Read the model definition and answer for the solid it produces. Units are mm, in the model's axes. A direction names the side the tool comes from. Coordinates: 2 decimals unless noted, no trailing zeros. Loops run counter-clockwise (first coordinate to the right, second up) from the corner with the lowest first, then second, coordinate; pieces in that order, holes last. Notation, with made-up numbers: (62.5, -2.5) -> (118.5, -2.5) arc R29 ccw to (118.5, 28.5) -> close; hole circle Ø2 at (67.25, 18.5). An arc over 180 degrees is marked (long way). Answer in a Markdown table with one row per item.
```python
from build123d import *

# Parameters (mm, degrees)
SKETCH_1_W           = 100
SKETCH_1_H           = 100
EXTRUDE_1_DEPTH      = 4
SKETCH_2_R           = 2.15
CUT_EXTRUDE_1_DEPTH  = 142.477913471
SKETCH_3_R           = 1.65
CUT_EXTRUDE_2_DEPTH  = 142.477913471
SKETCH_4_R           = 1.65
CUT_EXTRUDE_3_DEPTH  = 142.477913471
SKETCH_5_W           = 20.5
SKETCH_5_H           = 41.5
CUT_EXTRUDE_4_DEPTH  = 10
SKETCH_6_W           = 55
SKETCH_6_H           = 100
CUT_EXTRUDE_5_DEPTH  = 10
FILLET_2_R           = 1.2
SKETCH_8_R           = 1.65
CUT_EXTRUDE_6_DEPTH  = 142.477913471
SKETCH_9_W           = 15.75
SKETCH_9_H           = 78.5
CUT_EXTRUDE_7_DEPTH  = 142.477913471
CUT_EXTRUDE_8_DEPTH  = 10
FILLET_5_R           = 3
SKETCH_11_W          = 29.25
SKETCH_11_H          = 14
CUT_EXTRUDE_9_DEPTH  = 10
FILLET_7_R           = 3
SKETCH_12_R          = 1.65
CUT_EXTRUDE_10_DEPTH = 10
FILLET_8_R           = 3
EXTRUDE_2_DEPTH      = 4
FILLET_9_R           = 5
CUT_EXTRUDE_11_DEPTH = 10
FILLET_10_R          = 1.7
SKETCH_15_R          = 1.65
CUT_EXTRUDE_12_DEPTH = 10
FILLET_11_R          = 5


with BuildPart() as part:
    # 草图1 → 凸台-拉伸1 (new body)
    with BuildSketch(Plane.XY):
        with Locations((50, -50)):
            Rectangle(SKETCH_1_W, SKETCH_1_H)
    extrude(amount=EXTRUDE_1_DEPTH)

    # 草图2 → 切除-拉伸1 (cut, through all)
    with BuildSketch(Plane.XY.offset(4)):
        with Locations((80, -66)):
            Circle(SKETCH_2_R)
        with Locations((90, -66)):
            Circle(SKETCH_2_R)
        with Locations((90, -18)):
            Circle(SKETCH_2_R)
        with Locations((80, -18)):
            Circle(SKETCH_2_R)
    extrude(amount=-CUT_EXTRUDE_1_DEPTH, mode=Mode.SUBTRACT)

    # 草图3 → 切除-拉伸2 (cut, through all)
    with BuildSketch(Plane.XY.offset(4)):
        with Locations((73, -95)):
            Circle(SKETCH_3_R)
        with Locations((73, -85)):
            Circle(SKETCH_3_R)
        with Locations((85, -85)):
            Circle(SKETCH_3_R)
        with Locations((85, -95)):
            Circle(SKETCH_3_R)
    extrude(amount=-CUT_EXTRUDE_2_DEPTH, mode=Mode.SUBTRACT)

    # 草图4 → 切除-拉伸3 (cut, through all)
    with BuildSketch(Plane.XY.offset(4)):
        with BuildLine():
            ThreePointArc((81, -100), (71.5, -90.5), (62, -100))
            Line((62, -100), (81, -100))
        make_face()
        with Locations((73, -95)):
            Circle(SKETCH_4_R, mode=Mode.SUBTRACT)
    extrude(amount=-CUT_EXTRUDE_3_DEPTH, mode=Mode.SUBTRACT)

    # 草图5 → 切除-拉伸4 (cut)
    with BuildSketch(Plane.XY.offset(4)):
        with Locations((85, -42)):
            Rectangle(SKETCH_5_W, SKETCH_5_H)
    extrude(amount=-CUT_EXTRUDE_4_DEPTH, mode=Mode.SUBTRACT)

    # 草图6 → 切除-拉伸5 (cut)
    with BuildSketch(Plane.XY.offset(4)):
        with Locations((27.5, -50)):
            Rectangle(SKETCH_6_W, SKETCH_6_H)
    extrude(amount=-CUT_EXTRUDE_5_DEPTH, mode=Mode.SUBTRACT)

    # 圆角2
    fillet_2_edges = [part.edges().sort_by_distance(p)[0] for p in [
        (95.25, -62.75, 2),
        (74.75, -62.75, 2),
        (74.75, -21.25, 2),
        (95.25, -21.25, 2),
    ]]
    fillet(fillet_2_edges, radius=FILLET_2_R)

    # 草图8 → 切除-拉伸6 (cut, through all)
    with BuildSketch(Plane.XY.offset(4)):
        with Locations((59, -85)):
            Circle(SKETCH_8_R)
    extrude(amount=-CUT_EXTRUDE_6_DEPTH, mode=Mode.SUBTRACT)

    # 草图9 → 切除-拉伸7 (cut, through all)
    with BuildSketch(Plane.XY.offset(4)):
        with BuildLine():
            Line((71.5, -90.5), (55, -90.5))
            Line((55, -90.5), (55, -100))
            Line((55, -100), (62, -100))
            ThreePointArc((62, -100), (64.782485579, -93.282485579), (71.5, -90.5))
        make_face()
        with Locations((62.875, -39.25)):
            Rectangle(SKETCH_9_W, SKETCH_9_H)
    extrude(amount=-CUT_EXTRUDE_7_DEPTH, mode=Mode.SUBTRACT)

    # 草图10 → 切除-拉伸8 (cut)
    with BuildSketch(Plane.XY.offset(4)):
        with BuildLine():
            Line((100, -87.5), (55, -87.5))
            Line((55, -87.5), (55, -90.5))
            Line((55, -90.5), (71.5, -90.5))
            ThreePointArc((71.5, -90.5), (78.217514421, -93.282485579), (81, -100))
            Line((81, -100), (100, -100))
            Line((100, -100), (100, -87.5))
        make_face()
    extrude(amount=-CUT_EXTRUDE_8_DEPTH, mode=Mode.SUBTRACT)

    # 圆角5
    fillet_5_edges = [part.edges().sort_by_distance(p)[0] for p in [
        (100, -87.5, 2),
        (55, -87.5, 2),
    ]]
    fillet(fillet_5_edges, radius=FILLET_5_R)

    # 草图11 → 切除-拉伸9 (cut)
    with BuildSketch(Plane.XY.offset(4)):
        with Locations((85.375, -7)):
            Rectangle(SKETCH_11_W, SKETCH_11_H)
    extrude(amount=-CUT_EXTRUDE_9_DEPTH, mode=Mode.SUBTRACT)

    # 圆角7
    fillet_7_edges = [part.edges().sort_by_distance(p)[0] for p in [
        (70.75, -14, 2),
        (100, -14, 2),
    ]]
    fillet(fillet_7_edges, radius=FILLET_7_R)

    # 草图12 → 切除-拉伸10 (cut)
    with BuildSketch(Plane.XY.offset(4)):
        with BuildLine():
            Line((64.339745962, -87.5), (81.660254038, -87.5))
            ThreePointArc((81.660254038, -87.5), (73, -82.5), (64.339745962, -87.5))
        make_face()
        with Locations((73, -85)):
            Circle(SKETCH_12_R, mode=Mode.SUBTRACT)
    extrude(amount=-CUT_EXTRUDE_10_DEPTH, mode=Mode.SUBTRACT)

    # 圆角8
    fillet_8_edges = [part.edges().sort_by_distance(p)[0] for p in [
        (64.339745962, -87.5, 2),
        (81.660254038, -87.5, 2),
    ]]
    fillet(fillet_8_edges, radius=FILLET_8_R)

    # 草图13 → 凸台-拉伸2 (add)
    with BuildSketch(Plane.XY.offset(4)):
        Polygon((70.75, -51.220199781), (55, -78.5), (70.75, -78.5), align=None)
    extrude(amount=-EXTRUDE_2_DEPTH)

    # 圆角9
    fillet_9_edges = [part.edges().sort_by_distance(p)[0] for p in [
        (55, -78.5, 2),
        (70.75, -51.220199781, 2),
    ]]
    fillet(fillet_9_edges, radius=FILLET_9_R)

    # 草图14 → 切除-拉伸11 (cut)
    with BuildSketch(Plane.XY.offset(4)):
        Polygon((72.044228634, -79.339745962), (72.044228634, -56.97853003), (59.133974596, -79.339745962), align=None)
    extrude(amount=-CUT_EXTRUDE_11_DEPTH, mode=Mode.SUBTRACT)

    # 圆角10
    fillet_10_edges = [part.edges().sort_by_distance(p)[0] for p in [
        (72.044228634, -79.339745962, 2),
        (59.133974596, -79.339745962, 2),
        (72.044228634, -56.97853003, 2),
    ]]
    fillet(fillet_10_edges, radius=FILLET_10_R)

    # 草图15 → 切除-拉伸12 (cut)
    # profile 1 of 4: a face of its own
    with BuildSketch(Plane(origin=(0, 0, 0), x_dir=(-1, 0, 0), z_dir=(0, 0, -1))):
        with BuildLine():
            Line((-59.474464586, -70.75), (-55.667552662, -70.75))
            Line((-55.667552662, -70.75), (-55.667552662, -49.880453819))
            Line((-55.667552662, -49.880453819), (-70.75, -49.880453819))
            ThreePointArc((-70.75, -49.880453819), (-70.579629131, -51.174549044), (-70.080127019, -52.380453819))
            Line((-70.080127019, -52.380453819), (-59.474464586, -70.75))
        make_face()
    # profile 2 of 4: a face of its own
    with BuildSketch(Plane(origin=(0, 0, 0), x_dir=(-1, 0, 0), z_dir=(0, 0, -1))):
        with BuildLine():
            Line((-41.658398954, -70.75), (-55.667552662, -70.75))
            Line((-55.667552662, -70.75), (-59.474464586, -70.75))
            Line((-59.474464586, -70.75), (-55.669872981, -77.339745962))
            ThreePointArc((-55.669872981, -77.339745962), (-55.170370869, -78.545650737), (-55, -79.839745962))
            Line((-55, -79.839745962), (-55, -84.5))
            ThreePointArc((-55, -84.5), (-55.878679656, -86.621320344), (-58, -87.5))
            Line((-58, -87.5), (-62.753049234, -87.5))
            ThreePointArc((-62.753049234, -87.5), (-64.068636263, -87.196151103), (-65.11773018, -86.346153846))
            ThreePointArc((-65.11773018, -86.346153846), (-73, -82.5), (-80.88226982, -86.346153846))
            ThreePointArc((-80.88226982, -86.346153846), (-81.931363737, -87.196151103), (-83.246950766, -87.5))
            Line((-83.246950766, -87.5), (-97, -87.5))
            ThreePointArc((-97, -87.5), (-99.121320344, -86.621320344), (-100, -84.5))
            Line((-100, -84.5), (-100, -90.078728051))
            Line((-100, -90.078728051), (-41.658398954, -90.078728051))
            Line((-41.658398954, -90.078728051), (-41.658398954, -70.75))
        make_face()
    # profile 3 of 4: a face of its own
    with BuildSketch(Plane(origin=(0, 0, 0), x_dir=(-1, 0, 0), z_dir=(0, 0, -1))):
        with BuildLine():
            Line((-55.669872981, -77.339745962), (-59.474464586, -70.75))
            Line((-59.474464586, -70.75), (-64.09326674, -70.75))
            Line((-64.09326674, -70.75), (-60.606217783, -76.789745962))
            ThreePointArc((-60.606217783, -76.789745962), (-60.606217783, -78.489745962), (-62.078460969, -79.339745962))
            Line((-62.078460969, -79.339745962), (-70.344228634, -79.339745962))
            ThreePointArc((-70.344228634, -79.339745962), (-71.546310162, -78.84182749), (-72.044228634, -77.639745962))
            Line((-72.044228634, -77.639745962), (-72.044228634, -70.75))
            Line((-72.044228634, -70.75), (-100, -70.75))
            Line((-100, -70.75), (-100, -84.5))
            ThreePointArc((-100, -84.5), (-99.121320344, -86.621320344), (-97, -87.5))
            Line((-97, -87.5), (-83.246950766, -87.5))
            ThreePointArc((-83.246950766, -87.5), (-81.931363737, -87.196151103), (-80.88226982, -86.346153846))
            ThreePointArc((-80.88226982, -86.346153846), (-73, -82.5), (-65.11773018, -86.346153846))
            ThreePointArc((-65.11773018, -86.346153846), (-64.068636263, -87.196151103), (-62.753049234, -87.5))
            Line((-62.753049234, -87.5), (-58, -87.5))
            ThreePointArc((-58, -87.5), (-55.878679656, -86.621320344), (-55, -84.5))
            Line((-55, -84.5), (-55, -79.839745962))
            ThreePointArc((-55, -79.839745962), (-55.170370869, -78.545650737), (-55.669872981, -77.339745962))
        make_face()
        with Locations((-85, -85)):
            Circle(SKETCH_15_R, mode=Mode.SUBTRACT)
        with Locations((-59, -85)):
            Circle(SKETCH_15_R, mode=Mode.SUBTRACT)
    # profile 4 of 4: a face of its own
    with BuildSketch(Plane(origin=(0, 0, 0), x_dir=(-1, 0, 0), z_dir=(0, 0, -1))):
        with BuildLine():
            Line((-64.09326674, -70.75), (-59.474464586, -70.75))
            Line((-59.474464586, -70.75), (-70.080127019, -52.380453819))
            ThreePointArc((-70.080127019, -52.380453819), (-70.579629131, -51.174549044), (-70.75, -49.880453819))
            Line((-70.75, -49.880453819), (-70.75, -61.672153114))
            ThreePointArc((-70.75, -61.672153114), (-69.677380797, -61.759266435), (-68.871985448, -62.473016403))
            Line((-68.871985448, -62.473016403), (-64.09326674, -70.75))
        make_face()
    extrude(amount=-CUT_EXTRUDE_12_DEPTH, mode=Mode.SUBTRACT)

    # 圆角11
    fillet_11_edges = [part.edges().sort_by_distance(p)[0] for p in [
        (70.75, -61.672153114, 2),
        (100, -70.75, 2),
        (72.044228634, -70.75, 2),
    ]]
    fillet(fillet_11_edges, radius=FILLET_11_R)


solid = part.part
```
1. A cutting plane is placed at A-A on y = -18. Give the vertices of the cut face in (x, z).
A:
| item | result |
|---|---|
| outline | (70.75, 0) -> (77.85, 0) -> (77.85, 4) -> (70.75, 4) -> close; (82.15, 0) -> (87.85, 0) -> (87.85, 4) -> (82.15, 4) -> close; (92.15, 0) -> (100, 0) -> (100, 4) -> (92.15, 4) -> close |
2. Find the intervals of material crossed by probe 1 along Y at (x, z) = (80, 2.6); probe 2 along X at (y, z) = (-55, 2.2); probe 3 along Y at (x, z) = (87, 1.85), in increasing order.
A:
| item | result |
|---|---|
| probe 1 | y = -70.75 to -68.15, -63.85 to -62.75, -21.25 to -20.15, -15.85 to -14 |
| probe 2 | x = 70.75 to 74.75, 95.25 to 100 |
| probe 3 | y = -70.75 to -62.75, -21.25 to -14 |
3. The mould has two halves that part along Y. Classify faces 1 (the cylindrical face through (98.57, -69.25, 2.03)), 2 (the cylindrical face through (71.61, -14.9, 1.97)), 3 (the flat face through (74, -44, 0)), 4 (the cylindrical face through (75.092, -21.611, 1.972)): pulls with the +Y half, pulls with the -Y half, needs draft (parallel to the pull), parting line crosses it, or undercut.
A:
| item | result |
|---|---|
| face 1 | pulls with the -Y half |
| face 2 | pulls with the +Y half |
| face 3 | needs draft |
| face 4 | undercut |
4. A cutting plane is placed at B-B on x = 85.5. Give the vertices of the cut face in (y, z), and give its area (3 significant figures).
A:
| item | result |
|---|---|
| outline | (-70.75, 0) -> (-62.75, 0) -> (-62.75, 4) -> (-70.75, 4) -> close; (-21.25, 0) -> (-14, 0) -> (-14, 4) -> (-21.25, 4) -> close |
| area | 61.0 mm2 |
5. A tool of negligible diameter and unlimited length cuts with its end or side. For faces 5 (the flat face through (74.75, -42, 2)), 6 (the cylindrical face through (99.1, -14.86, 1.97)), 7 (the flat face through (72.044, -65, 2)), from which of +Z, -Z, +X, -X, +Y, -Y can it reach the whole face along a straight path? Write none if from no direction.
A:
| item | result |
|---|---|
| face 5 | +Z, -Z |
| face 6 | +Z, -Z, +X, +Y |
| face 7 | +Z, -Z, -X, -Y |
6. A cutting plane is placed at C-C on x = 90. Give the vertices of the cut face in (y, z).
A:
| item | result |
|---|---|
| outline | (-70.75, 0) -> (-68.15, 0) -> (-68.15, 4) -> (-70.75, 4) -> close; (-63.85, 0) -> (-62.75, 0) -> (-62.75, 4) -> (-63.85, 4) -> close; (-21.25, 0) -> (-20.15, 0) -> (-20.15, 4) -> (-21.25, 4) -> close; (-15.85, 0) -> (-14, 0) -> (-14, 4) -> (-15.85, 4) -> close |
7. A cutting plane is placed at D-D on y = -51. Give the vertices of the cut face in (x, z), and give its area (3 significant figures).
A:
| item | result |
|---|---|
| outline | (70.75, 0) -> (74.75, 0) -> (74.75, 4) -> (70.75, 4) -> close; (95.25, 0) -> (100, 0) -> (100, 4) -> (95.25, 4) -> close |
| area | 35.0 mm2 |
